from build123d import *

# Parameters (mm, degrees)
SKETCH1_R           = 90
BOSS_EXTRUDE1_DEPTH = 15
SKETCH2_R           = 12.5
CUT_EXTRUDE1_DEPTH  = 129.16005618
SKETCH3_R           = 8.190815025
CUT_EXTRUDE2_DEPTH  = 14.661514
CIRPATTERN1_START   = 0.33848578
CIRPATTERN1_DEPTH   = 14.66151422


# Read off the part's stored shape, not the designer's step: CirPattern1
with BuildPart() as part:
    # Sketch1 → Boss-Extrude1 (new body)
    with BuildSketch(Plane(origin=(0, 0, 0), x_dir=(1, 0, 0), z_dir=(0, 1, 0))):
        with Locations(Location((0, 0, 0), (0, 0, 270))):
            Circle(SKETCH1_R)
    extrude(amount=BOSS_EXTRUDE1_DEPTH)

    # Sketch2 → Cut-Extrude1 (cut, through all)
    with BuildSketch(Plane(origin=(0, 0, 0), x_dir=(1, 0, 0), z_dir=(0, 1, 0))):
        with Locations(Location((0, 0, 0), (0, 0, 270))):
            Circle(SKETCH2_R)
    extrude(amount=CUT_EXTRUDE1_DEPTH, mode=Mode.SUBTRACT)

    # Sketch3 → Cut-Extrude2 (cut)
    with BuildSketch(Plane(origin=(0, 15, 0), x_dir=(1, 0, 0), z_dir=(0, 1, 0))):
        with Locations((-11.303338173, 0)):
            Circle(SKETCH3_R)
    extrude(amount=-CUT_EXTRUDE2_DEPTH, mode=Mode.SUBTRACT)

    # CirPattern1 outline → CirPattern1 (cut)
    with BuildSketch(Plane(origin=(0, 0, 0), x_dir=(1, 0, 0), z_dir=(0, 1, 0)).offset(CIRPATTERN1_START)):
        with BuildLine():
            ThreePointArc((-9.595661024, -8.010823274), (-11.613203912, -8.18495168), (-13.611806453, -7.85878012))
            ThreePointArc((-13.611806453, -7.85878012), (-9.747076599, -16.882431895), (0, -15.717560239))
            ThreePointArc((0, -15.717560239), (9.747076599, -16.882431895), (13.611806453, -7.85878012))
            ThreePointArc((13.611806453, -7.85878012), (19.494153198, 0), (13.611806453, 7.85878012))
            ThreePointArc((13.611806453, 7.85878012), (9.747076599, 16.882431895), (0, 15.717560239))
            ThreePointArc((0, 15.717560239), (-9.747076599, 16.882431895), (-13.611806453, 7.85878012))
            ThreePointArc((-13.611806453, 7.85878012), (-11.613203912, 8.18495168), (-9.595661024, 8.010823274))
            ThreePointArc((-9.595661024, 8.010823274), (12.5, 0), (-9.595661024, -8.010823274))
        make_face()
    extrude(amount=CIRPATTERN1_DEPTH, mode=Mode.SUBTRACT)


solid = part.part
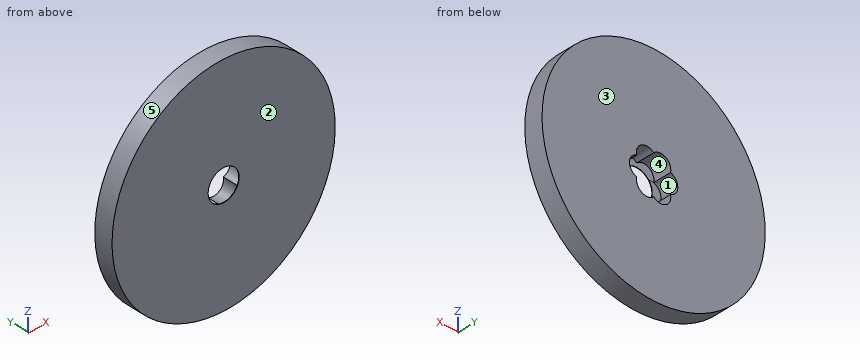
Part model, mm, in its own coordinate system. Face numbers are marked on the shaded views. A direction names the side the tool comes from. Round coordinates to 2 decimals unless told otherwise and drop trailing zeros. Write each loop counter-clockwise with the first axis right and the second up, starting at its lowest first coordinate (ties: lowest second). Pieces come first, ordered by that corner, then holes. Notation, with made-up numbers: M -15.5,85.5 L 42.5,85.5 A19 ccw 42.5,99.5 Z; hole C -31.75,-21.75 d8. An arc over 180 degrees is marked long. Return JSON: item names as keys, results as strings. Group by question number.
(1) Saw through at A-A on z = 0. Write the cut outline in (x, y), then the cut area to 3 significant figures.
(2) Which spindle directions (+Z, -Z, +X, -X, +Y, -Y) get a long thin tool onto all of the face, cutting with end or side? Do the marked faces 1 and 2. Say none if no direction does.
(3) Saw through at B-B on y = 8. Write the cut outline in (x, z), then the cut area to 3 significant figures.
(4) Two-plate mould, pull along X, no slides. Class the marked faces 3, 4 and 5: +X half, -X half, draft (parallel to the pull), parting line (faces both ways), or undercut.
(5) Saw through at D-D on x = -31.5. Write the cut outline in (y, z), then the cut area to 3 significant figures.
(6) Pin check, flat tips, straight feed: pin 1 Ø6 at (y, z) = (4.5, 52.5) entering from +X; pin 2 Ø8 at (x, y) = (13.5, 2) entering from +Z; pin 3 Ø4 at (y, z) = (10.5, 63.5) entering from -X. Stop position of each tip, or through.
(7) Drill centre lines: probe 1 along X at (y, z) = (0.25, 0); probe 2 along Z at (x, y) = (5, 11.25); probe 3 along X at (y, z) = (7, -6.5). Where is each one in solid material? Low to high.
(8) Saw through at C-C on x = 6.5. Write the cut outline in (y, z), then the cut area to 3 significant figures.
Returned:
{
 "1": {"outline": "M -90,0 L -12.5,0 L -12.5,0.34 L -19.49,0.34 L -19.49,15 L -90,15 Z; M 12.5,0 L 90,0 L 90,15 L 19.49,15 L 19.49,0.34 L 12.5,0.34 Z", "area": "2,120 mm²"},
 "2": {"face 1": "+Y", "face 2": "+Z, -Z, +X, -X, -Y"},
 "3": {"outline": "C 0,0 d180; hole M -13.61,-7.86 A8.19 ccw 0,-15.72 A8.19 ccw 13.61,-7.86 A8.19 ccw 13.61,7.86 A8.19 ccw 0,15.72 A8.19 ccw -13.61,7.86 A8.19 ccw Z", "area": "24,400 mm²"},
 "4": {"face 3": "draft", "face 4": "undercut", "face 5": "parting line"},
 "5": {"outline": "M 0,-84.31 L 15,-84.31 L 15,84.31 L 0,84.31 Z", "area": "2,530 mm²"},
 "6": {"pin 1": "x = 75.16", "pin 2": "z = 89.5", "pin 3": "x = -65.71"},
 "7": {"probe 1": "-90 to -12.5, 12.5 to 90", "probe 2": "-89.86 to -17.95, 17.95 to 89.86", "probe 3": "-89.76 to -16.29, 16.29 to 89.76"},
 "8": {"outline": "M 0,-89.76 L 15,-89.76 L 15,-17.94 L 0.34,-17.94 L 0.34,-10.68 L 0,-10.68 Z; M 0,10.68 L 0.34,10.68 L 0.34,17.94 L 15,17.94 L 15,89.76 L 0,89.76 Z", "area": "2,160 mm²"}
}
